For this review, use the dimensioned drawing (mm, ordinates from the lowest corner) and the shaded views. A direction names the side the tool comes from. Give positions to 0.01 mm unless a question says otherwise; leave off trailing zeros. Loops run counter-clockwise (first coordinate to the right, second up) from the corner with the lowest first, then second, coordinate; pieces in that order, holes last. Notation, with made-up numbers: M 59.5,64 L 118.5,64 A36 ccw 118.5,101 Z; hole C 51.25,-31 d8. An arc over 180 degrees is marked long. Use CSV: the item, a comma, the result in double quotes. Start each with the question number.
1. Take a section at A-A, the plane y = 47.5. Write out the cut boundary in (x, z).
2. Insertion check: P1, Ø6.5, axis at x = 24, y = 47.5, coming from the -Z side; P2, Ø0.8, axis at x = 96.5, y = 93.5, coming from the +Z side; P3, Ø2, axis at x = 76, y = 14, coming from the +Z side. Each pin has a flat end and moves straight along its axis. Give the tip position at first contact, or say it passes through.
3. Take a section at D-D, the plane x = 65. Write out the cut boundary in (y, z).
4. To check wall thickness, follow line 1 (X direction, y = 47, z = 1); line 2 (X direction, y = 6.5, z = 40.5); line 3 (Y direction, x = 136, z = 1). State the ranges of each line that lie inside material, in increasing order. Write a range as [from, to].
5. The part is to be moulded in two halves that separate along Y. For the marked faces 1, 2, 3 and 4, say which applies: pulls with the +Y half, pulls with the -Y half, needs draft (parallel to the pull), parting line crosses it, or undercut.
6. Take a section at C-C, the plane x = 24. Write out the cut boundary in (y, z), and give its area (3 significant figures).
7. Take a section at B-B, the plane z = 62. Write out the cut boundary in (x, y).
8. Tool access review of the marked faces 5 and 6: name each direction out of +Z, -Z, +X, -X, +Y, -Y from which nothing blocks a thin tool from reaching the whole face with its end or side.
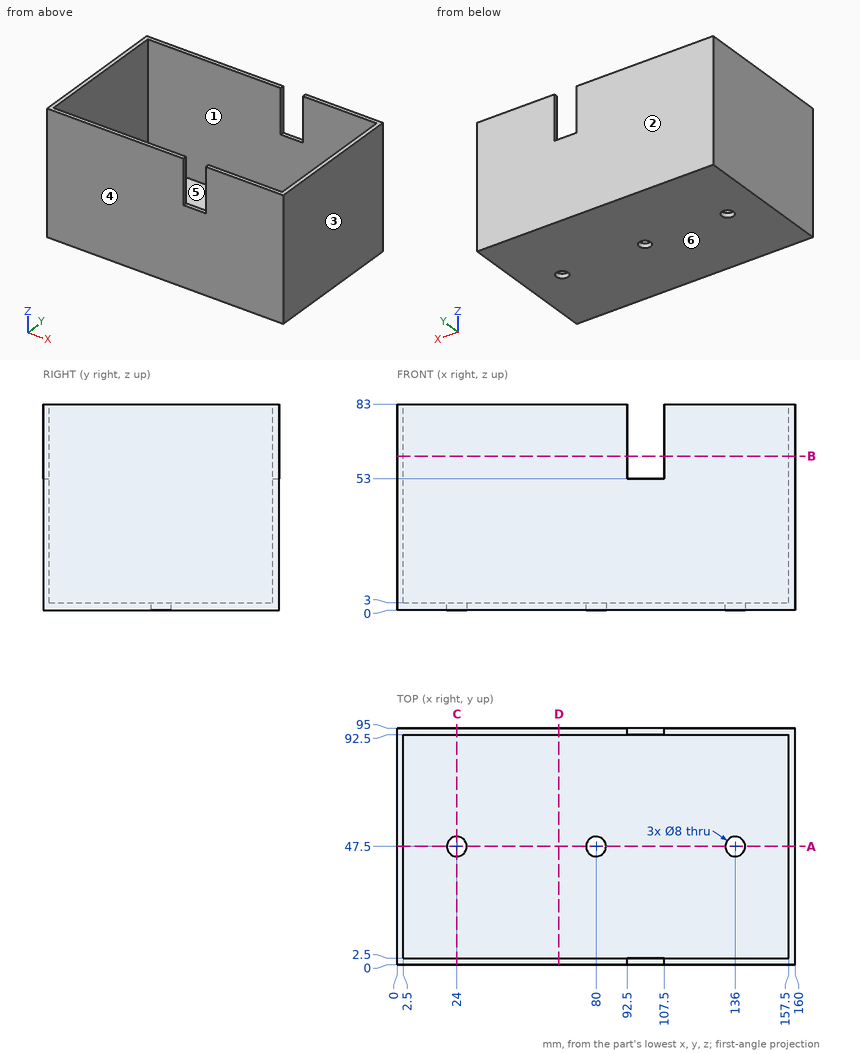
Result set:
1,outline,"M 0,0 L 20,0 L 20,3 L 2.5,3 L 2.5,83 L 0,83 Z; M 28,0 L 76,0 L 76,3 L 28,3 Z; M 84,0 L 132,0 L 132,3 L 84,3 Z; M 140,0 L 160,0 L 160,83 L 157.5,83 L 157.5,3 L 140,3 Z"
2,P1,"through"
2,P2,"z = 53"
2,P3,"z = 3"
3,outline,"M 0,0 L 95,0 L 95,83 L 92.5,83 L 92.5,3 L 2.5,3 L 2.5,83 L 0,83 Z"
4,line 1,"[0, 20.03], [27.97, 76.03], [83.97, 132.03], [139.97, 160]"
4,line 2,"[0, 2.5], [157.5, 160]"
4,line 3,"[0, 43.5], [51.5, 95]"
5,face 1,"undercut"
5,face 2,"pulls with the +Y half"
5,face 3,"needs draft"
5,face 4,"pulls with the -Y half"
6,outline,"M 0,0 L 43.5,0 L 43.5,3 L 2.5,3 L 2.5,83 L 0,83 Z; M 51.5,0 L 95,0 L 95,83 L 92.5,83 L 92.5,3 L 51.5,3 Z"
6,area,"661 mm2"
7,outline,"M 0,0 L 92.5,0 L 92.5,2.5 L 2.5,2.5 L 2.5,92.5 L 92.5,92.5 L 92.5,95 L 0,95 Z; M 107.5,0 L 160,0 L 160,95 L 107.5,95 L 107.5,92.5 L 157.5,92.5 L 157.5,2.5 L 107.5,2.5 Z"
8,face 5,"+Z"
8,face 6,"-Z, +X, -X, +Y, -Y"
